Geometry check sheet. Reference: the model listing, model coordinates, mm. Face numbers are marked on the shaded views. A direction names the side the tool comes from. Round coordinates to 2 decimals unless told otherwise and drop trailing zeros. Write each loop counter-clockwise with the first axis right and the second up, starting at its lowest first coordinate (ties: lowest second). Pieces come first, ordered by that corner, then holes. Notation, with made-up numbers: (47.25, -35.75) -> (73.25, -35.75) arc R16 cw to (73.25, -20.75) -> close; hole circle Ø9 at (27, -14.5). An arc over 180 degrees is marked (long way). One line per question, with ' | ' between items.
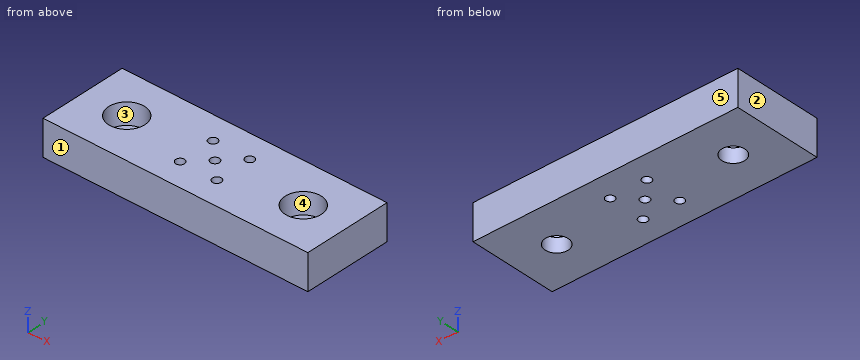
```python
from build123d import *

# Parameters (mm, degrees)
SKETCH1_R           = 3.25
SKETCH1_R_2         = 1.25
BOSS_EXTRUDE1_DEPTH = 10
SKETCH2_R           = 5.11
CUT_EXTRUDE1_DEPTH  = 6


with BuildPart() as part:
    # Sketch1 → Boss-Extrude1 (new body)
    with BuildSketch(Plane.XY):
        Polygon((-37.5, 12.5), (37.5, 12.5), (37.5, 0), (37.5, -12.5), (-37.5, -12.5), (-37.5, 0), align=None)
        with Locations((-25, 0)):
            Circle(SKETCH1_R, mode=Mode.SUBTRACT)
        with Locations((25, 0)):
            Circle(SKETCH1_R, mode=Mode.SUBTRACT)
        Circle(SKETCH1_R_2, mode=Mode.SUBTRACT)
        with Locations((-5.2, 5.2)):
            Circle(SKETCH1_R_2, mode=Mode.SUBTRACT)
        with Locations((5.2, 5.2)):
            Circle(SKETCH1_R_2, mode=Mode.SUBTRACT)
        with Locations((5.2, -5.2)):
            Circle(SKETCH1_R_2, mode=Mode.SUBTRACT)
        with Locations((-5.2, -5.2)):
            Circle(SKETCH1_R_2, mode=Mode.SUBTRACT)
    extrude(amount=BOSS_EXTRUDE1_DEPTH)

    # Sketch2 → Cut-Extrude1 (cut)
    with BuildSketch(Plane.XY.offset(10)):
        with Locations((-25, 0)):
            Circle(SKETCH2_R)
        with Locations((25, 0)):
            Circle(SKETCH2_R)
    extrude(amount=-CUT_EXTRUDE1_DEPTH, mode=Mode.SUBTRACT)


solid = part.part
```
(1) Sectioned sample at C-C on y = 0. Record the cut outline in (x, z).
Resolved:
outline: (-37.5, 0) -> (-28.25, 0) -> (-28.25, 4) -> (-30.11, 4) -> (-30.11, 10) -> (-37.5, 10) -> close; (-21.75, 0) -> (-1.25, 0) -> (-1.25, 10) -> (-19.89, 10) -> (-19.89, 4) -> (-21.75, 4) -> close; (1.25, 0) -> (21.75, 0) -> (21.75, 4) -> (19.89, 4) -> (19.89, 10) -> (1.25, 10) -> close; (28.25, 0) -> (37.5, 0) -> (37.5, 10) -> (30.11, 10) -> (30.11, 4) -> (28.25, 4) -> close
(2) Material ranges on line 1 (Y direction, x = 5.2, z = 5.5); line 2 (Y direction, x = -25, z = 2.4); line 3 (X direction, y = 2, z = 6), recorded low to high.
Resolved:
line 1: y = -12.5 to -6.45, -3.95 to 3.95, 6.45 to 12.5 | line 2: y = -12.5 to -3.25, 3.25 to 12.5 | line 3: x = -37.5 to -29.7, -20.3 to 20.3, 29.7 to 37.5
(3) Sectioned sample at D-D on z = 5. Record the cut outline in (x, y), then the cut area to 3 significant figures.
Resolved:
outline: (-37.5, -12.5) -> (37.5, -12.5) -> (37.5, 12.5) -> (-37.5, 12.5) -> close; hole circle Ø10.22 at (-25, 0); hole circle Ø2.5 at (-5.2, -5.2); hole circle Ø2.5 at (-5.2, 5.2); hole circle Ø2.5 at (0, 0); hole circle Ø2.5 at (5.2, -5.2); hole circle Ø2.5 at (5.2, 5.2); hole circle Ø10.22 at (25, 0) | area: 1,690 mm2
(4) Draft check along Y on the marked faces 1, 2 and 3. Enter one of: +Y half, -Y half, draft (parallel to the pull), parting line (faces both ways), or undercut.
Resolved:
face 1: -Y half | face 2: draft | face 3: undercut
(5) Access from +Z, -Z, +X, -X, +Y, -Y to the whole of each face (thin tool, end or side, straight path). Record for the marked faces 4 and 5.
Resolved:
face 4: +Z | face 5: +Z, -Z, +X, -X, +Y
(6) Go/stop test with flat-tipped pins: pin 1 (2 mm diameter, centred on x = 5.2, y = -5.2, fed in from -Z); pin 2 (5 mm diameter, centred on x = 24, y = 2, fed in from +Z). Record where each tip stops, or that it passes through.
Resolved:
pin 1: passes through | pin 2: stops at z = 4
(7) Sectioned sample at B-B on z = 1.5. Record the cut outline in (x, y), then the cut area to 3 significant figures.
Resolved:
outline: (-37.5, -12.5) -> (37.5, -12.5) -> (37.5, 12.5) -> (-37.5, 12.5) -> close; hole circle Ø6.5 at (-25, 0); hole circle Ø2.5 at (-5.2, -5.2); hole circle Ø2.5 at (-5.2, 5.2); hole circle Ø2.5 at (0, 0); hole circle Ø2.5 at (5.2, -5.2); hole circle Ø2.5 at (5.2, 5.2); hole circle Ø6.5 at (25, 0) | area: 1,780 mm2
(8) Sectioned sample at A-A on x = 0. Record the cut outline in (y, z), then the cut area to 3 significant figures.
Resolved:
outline: (-12.5, 0) -> (-1.25, 0) -> (-1.25, 10) -> (-12.5, 10) -> close; (1.25, 0) -> (12.5, 0) -> (12.5, 10) -> (1.25, 10) -> close | area: 225 mm2
